from build123d import *

# Parameters (mm, degrees)
SKETCH1_W                    = 11.684
SKETCH1_H                    = 1.5875
F_36_0_1065_DIAMETER_HOLE1_D = 2.7051
SCREW_PASSTHROUGHS_COUNT     = 12


with BuildPart() as part:
    # Sketch1 → Main (revolve)
    with BuildSketch(Plane.XY):
        with Locations((-43.942, 0.79375)):
            Rectangle(SKETCH1_W, SKETCH1_H)
    revolve(axis=Axis((0, 55, 0), (0, -1, 0)))

    # #36 (0.1065) Diameter Hole1 (through all)
    with Locations(Plane(origin=(0, 0, 0), x_dir=(-1, 0, 0), z_dir=(0, -1, 0))):
        with Locations((45.6057, 0)):
            f_36_0_1065_diameter_hole1 = Hole(F_36_0_1065_DIAMETER_HOLE1_D / 2)

    # Screw Passthroughs: #36 (0.1065) Diameter Hole1 ×12 about axis
    screw_passthroughs_axis = Axis((0, 0, 0), (0, 1, 0))
    for i in range(1, SCREW_PASSTHROUGHS_COUNT):
        add(f_36_0_1065_diameter_hole1.rotate(screw_passthroughs_axis, i * 360 / SCREW_PASSTHROUGHS_COUNT), mode=Mode.SUBTRACT)


solid = part.part
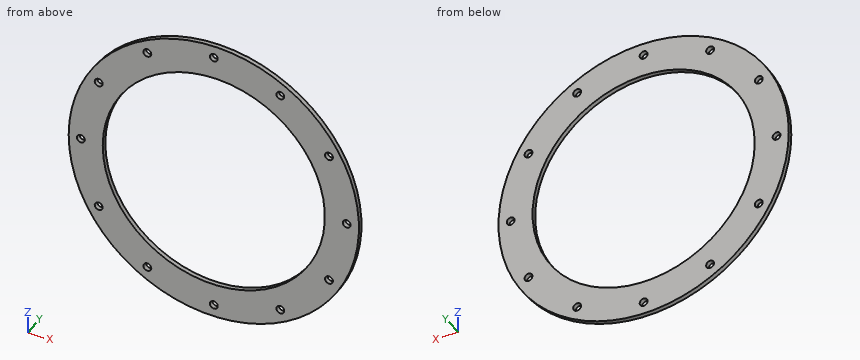
For this review, take the finished solid that the model builds, in its own axes (mm). Give positions to 0.01 mm unless a question says otherwise; leave off trailing zeros. Loops run counter-clockwise (first coordinate to the right, second up) from the corner with the lowest first, then second, coordinate; pieces in that order, holes last. Notation, with made-up numbers: M -25,41.5 L 5,41.5 A14 ccw 5,68.5 Z; hole C 7.25,-16 d6. An arc over 180 degrees is marked long. Answer as a JSON object with one key per item and string values. Group by question number.
Q1. Add section D-D on z = 19.5. Give the boundary of the cut face in (x, y), and give its area (3 significant figures).
Q2. Add section B-B on z = 0. Give the boundary of the cut face in (x, y), and give its area (3 significant figures).
Q3. For probe 1 along Z at (x, y) = (39, 1.35); probe 2 along Z at (x, y) = (-38.5, 0.15); probe 3 along X at (y, z) = (1.4, 1) (3 decimals), list the stretches that pass through material, from the lowest coordinate up. Write a range as [from, to].
Q4. Insertion check: P1, Ø5, axis at x = 36, z = -28, coming from the -Y side; P2, Ø1.6, axis at x = 22.8, z = -39.5, coming from the -Y side. Each pin has a flat end and moves straight along its axis. Give the tip position at first contact, or say it passes through.
Q5. Add section C-C on x = -14. Give the boundary of the cut face in (y, z).
Q6. Add section A-A on x = 0. Give the boundary of the cut face in (y, z), and give its area (3 significant figures).
Checked values:
{
 "1": {"outline": "M -45.81,0 L -32.73,0 L -32.73,1.59 L -45.81,1.59 Z; M 32.73,0 L 45.81,0 L 45.81,1.59 L 32.73,1.59 Z", "area": "41.5 mm²"},
 "2": {"outline": "M -49.78,0 L -46.96,0 L -46.96,1.59 L -49.78,1.59 Z; M -44.25,0 L -38.1,0 L -38.1,1.59 L -44.25,1.59 Z; M 38.1,0 L 44.25,0 L 44.25,1.59 L 38.1,1.59 Z; M 46.96,0 L 49.78,0 L 49.78,1.59 L 46.96,1.59 Z", "area": "28.5 mm²"},
 "3": {"probe 1": "[-30.94, -24.06], [-21.54, 21.54], [24.06, 30.94]", "probe 2": "[-31.56, -23.72], [-21.89, 21.89], [23.72, 31.56]", "probe 3": "[-49.774, -46.516], [-44.695, -38.087], [38.087, 44.695], [46.516, 49.774]"},
 "4": {"P1": "y = 0", "P2": "through"},
 "5": {"outline": "M 0,-47.77 L 1.59,-47.77 L 1.59,-35.43 L 0,-35.43 Z; M 0,35.43 L 1.59,35.43 L 1.59,47.77 L 0,47.77 Z"},
 "6": {"outline": "M 0,-49.78 L 1.59,-49.78 L 1.59,-46.96 L 0,-46.96 Z; M 0,-44.25 L 1.59,-44.25 L 1.59,-38.1 L 0,-38.1 Z; M 0,38.1 L 1.59,38.1 L 1.59,44.25 L 0,44.25 Z; M 0,46.96 L 1.59,46.96 L 1.59,49.78 L 0,49.78 Z", "area": "28.5 mm²"}
}
